Work out the finished part from the listing and answer in its coordinate system (mm). Round coordinates to 2 decimals unless told otherwise and drop trailing zeros. Write each loop counter-clockwise with the first axis right and the second up, starting at its lowest first coordinate (ties: lowest second). Pieces come first, ordered by that corner, then holes. Notation, with made-up numbers: (74.25, -30.5) -> (124.25, -30.5) arc R12 cw to (124.25, -14.5) -> close; hole circle Ø9 at (2.25, 60.5). An arc over 180 degrees is marked (long way). One line per item, written item: value.
```python
from build123d import *

# Parameters (mm, degrees)
SKETCH1_R           = 15
BOSS_EXTRUDE1_DEPTH = 10


with BuildPart() as part:
    # Sketch1 → Boss-Extrude1 (new body)
    with BuildSketch(Plane(origin=(0, 0, 0), x_dir=(1, 0, 0), z_dir=(0, 1, 0))):
        with BuildLine():
            Line((-370, -100), (370, -100))
            ThreePointArc((370, -100), (391.213203436, -91.213203436), (400, -70))
            Line((400, -70), (400, 70))
            ThreePointArc((400, 70), (391.213203436, 91.213203436), (370, 100))
            Line((370, 100), (44.619962618, 100))
            ThreePointArc((44.619962618, 100), (66.975731412, 73.469642109), (75, 39.716843679))
            ThreePointArc((75, 39.716843679), (-33.75279843, -27.258887733), (-44.619962618, 100))
            Line((-44.619962618, 100), (-370, 100))
            ThreePointArc((-370, 100), (-391.213203436, 91.213203436), (-400, 70))
            Line((-400, 70), (-400, -70))
            ThreePointArc((-400, -70), (-391.213203436, -91.213203436), (-370, -100))
        make_face()
        with Locations(Location((-300.6181604, -75.1545401, 0), (0, 0, 270))):
            Circle(SKETCH1_R, mode=Mode.SUBTRACT)
        with Locations(Location((-92.979550381, -75.1545401, 0), (0, 0, 270))):
            Circle(SKETCH1_R, mode=Mode.SUBTRACT)
        with Locations(Location((92.979550381, -75.1545401, 0), (0, 0, 270))):
            Circle(SKETCH1_R, mode=Mode.SUBTRACT)
        with Locations(Location((300.6181604, -75.1545401, 0), (0, 0, 270))):
            Circle(SKETCH1_R, mode=Mode.SUBTRACT)
        with Locations(Location((-370, 24.949199623, 0), (0, 0, 270))):
            Circle(SKETCH1_R, mode=Mode.SUBTRACT)
        with Locations(Location((-182.623487934, 24.949199623, 0), (0, 0, 270))):
            Circle(SKETCH1_R, mode=Mode.SUBTRACT)
        with BuildLine():
            ThreePointArc((-242.623487934, 76.468107678), (-239.694555745, 83.53917549), (-232.623487934, 86.468107678))
            Line((-232.623487934, 86.468107678), (-192.623487934, 86.468107678))
            ThreePointArc((-192.623487934, 86.468107678), (-185.552420122, 83.53917549), (-182.623487934, 76.468107678))
            Line((-182.623487934, 76.468107678), (-182.623487934, 66.468107678))
            ThreePointArc((-182.623487934, 66.468107678), (-185.552420122, 59.397039866), (-192.623487934, 56.468107678))
            Line((-192.623487934, 56.468107678), (-232.623487934, 56.468107678))
            ThreePointArc((-232.623487934, 56.468107678), (-239.694555745, 59.397039866), (-242.623487934, 66.468107678))
            Line((-242.623487934, 66.468107678), (-242.623487934, 76.468107678))
        make_face(mode=Mode.SUBTRACT)
        with Locations(Location((182.623487934, 24.949199623, 0), (0, 0, 270))):
            Circle(SKETCH1_R, mode=Mode.SUBTRACT)
        with Locations(Location((370, 24.949199623, 0), (0, 0, 270))):
            Circle(SKETCH1_R, mode=Mode.SUBTRACT)
        with BuildLine():
            ThreePointArc((242.623487934, 66.468107678), (239.694555745, 59.397039866), (232.623487934, 56.468107678))
            Line((232.623487934, 56.468107678), (192.623487934, 56.468107678))
            ThreePointArc((192.623487934, 56.468107678), (185.552420122, 59.397039866), (182.623487934, 66.468107678))
            Line((182.623487934, 66.468107678), (182.623487934, 76.468107678))
            ThreePointArc((182.623487934, 76.468107678), (185.552420122, 83.53917549), (192.623487934, 86.468107678))
            Line((192.623487934, 86.468107678), (232.623487934, 86.468107678))
            ThreePointArc((232.623487934, 86.468107678), (239.694555745, 83.53917549), (242.623487934, 76.468107678))
            Line((242.623487934, 76.468107678), (242.623487934, 66.468107678))
        make_face(mode=Mode.SUBTRACT)
    extrude(amount=BOSS_EXTRUDE1_DEPTH)


solid = part.part
```
(1) For a pull along Z with two mould halves and no side action, classify faces 1 (the face through (-6, 0, 43)), 2 (the face through (391.445, 4.93, -90.979)), 3 (the face through (-80.331, 4.93, 83.218)) as pulls with the +Z half, pulls with the -Z half, needs draft (parallel to the pull), parting line crosses it, or undercut.
Reported:
face 1: needs draft
face 2: pulls with the -Z half
face 3: undercut
(2) Find section A-A on x = 0. Give the vertices of the cut face in (y, z), plus the area to 3 significant figures.
Reported:
outline: (0, 35.28) -> (10, 35.28) -> (10, 100) -> (0, 100) -> close
area: 647 mm2
(3) Consider probe 1 along Z at (x, y) = (-222.5, 1.25); probe 2 along X at (y, z) = (6.5, -73); probe 3 along X at (y, z) = (7, -30.5). Determine where each line is inside the solid, lowest interval first.
Reported:
probe 1: z = -100 to -86.47, -56.47 to 100
probe 2: x = -399.85 to -242.62, -182.62 to -67.21, 67.21 to 182.62, 242.62 to 399.85
probe 3: x = -400 to -383.94, -356.06 to -196.56, -168.69 to -74.43, 74.43 to 168.69, 196.56 to 356.06, 383.94 to 400
